Verification items for the finished model (mm, model axes). Face numbers are marked on the shaded views. A direction names the side the tool comes from. Round coordinates to 2 decimals unless told otherwise and drop trailing zeros. Write each loop counter-clockwise with the first axis right and the second up, starting at its lowest first coordinate (ties: lowest second). Pieces come first, ordered by that corner, then holes. Notation, with made-up numbers: (73, -29.75) - (129, -29.75) arc R16 ccw to (129, -18.75) - close; hole circle Ø8 at (-3, 11.25). An arc over 180 degrees is marked (long way). Answer as a JSON object with one key per item and string values. Group by question number.
1) Thickness scan on line 1 (X direction, y = 47, z = 80.5); line 2 (Y direction, x = 23, z = 63.5). Record the ranges inside material, lowest first.
2) Section check C-C (z = 52). Enter the section's corners in (x, y), then the cut area to 3 significant figures.
3) Section check B-B (y = 39.5). Enter the section's corners in (x, z), then the cut area to 3 significant figures.
4) Section check D-D (z = 25). Enter the section's corners in (x, y).
5) Section check A-A (x = 19.19). Enter the section's corners in (y, z).
6) Go/stop test with flat-tipped pins: pin 1 Ø4 at (x, z) = (2.5, 60.5) entering from -Y; pin 2 Ø6.5 at (x, z) = (47, 66.5) entering from -Y; pin 3 Ø3 at (x, y) = (46.5, -3.5) entering from -Z. Record where each tip stops, or that it passes through.
7) Set-up check for the marked faces 1 and 2: record each of +Z, -Z, +X, -X, +Y, -Y from which the full face is reachable in a straight line by a thin tool's end or side.
8) Mould release check, pull along X, two halves, no side actions. Record for the marked faces 3, 4 and 5: +X half, -X half, draft (parallel to the pull), parting line (faces both ways), or undercut.
```python
from build123d import *

# Parameters (mm, degrees)
BOSS_EXTRUDE1_DEPTH = 120
SKETCH2_W           = 20
SKETCH2_H           = 6
BOSS_EXTRUDE2_DEPTH = 6
SKETCH3_W           = 20
SKETCH3_H           = 6
BOSS_EXTRUDE3_DEPTH = 6
SKETCH4_R           = 1.6
CUT_EXTRUDE1_DEPTH  = 10


with BuildPart() as part:
    # Sketch1 → Boss-Extrude1 (new body)
    with BuildSketch(Plane.XY):
        Polygon((42.5, 0), (42.5, 50), (-42.5, 50), (-42.5, 0), (-48.5, 0), (-48.5, 56), (48.5, 56), (48.5, 0), align=None)
    extrude(amount=BOSS_EXTRUDE1_DEPTH)

    # Sketch2 → Boss-Extrude2 (add)
    with BuildSketch(Plane(origin=(48.5, 0, 0), x_dir=(0, 0, -1), z_dir=(1, 0, 0))):
        with Locations((-90, -3)):
            Rectangle(SKETCH2_W, SKETCH2_H)
        with Locations((-30, -3)):
            Rectangle(SKETCH2_W, SKETCH2_H)
    extrude(amount=-BOSS_EXTRUDE2_DEPTH)

    # Sketch3 → Boss-Extrude3 (add)
    with BuildSketch(Plane.ZY.offset(48.5)):
        with Locations((30, -3)):
            Rectangle(SKETCH3_W, SKETCH3_H)
        with Locations((90, -3)):
            Rectangle(SKETCH3_W, SKETCH3_H)
    extrude(amount=-BOSS_EXTRUDE3_DEPTH)

    # Sketch4 → Cut-Extrude1 (cut)
    with BuildSketch(Plane(origin=(0, 56, 0), x_dir=(1, 0, 0), z_dir=(0, 1, 0))):
        with Locations(Location((-23.905, -86.79842215, 0), (0, 0, 270))):
            Circle(SKETCH4_R)
        with Locations(Location((23.905, -86.79842215, 0), (0, 0, 270))):
            Circle(SKETCH4_R)
        with Locations(Location((-8.71, -35.65842215, 0), (0, 0, 270))):
            Circle(SKETCH4_R)
        with Locations(Location((19.19, -35.65842215, 0), (0, 0, 270))):
            Circle(SKETCH4_R)
    extrude(amount=-CUT_EXTRUDE1_DEPTH, mode=Mode.SUBTRACT)


solid = part.part
```
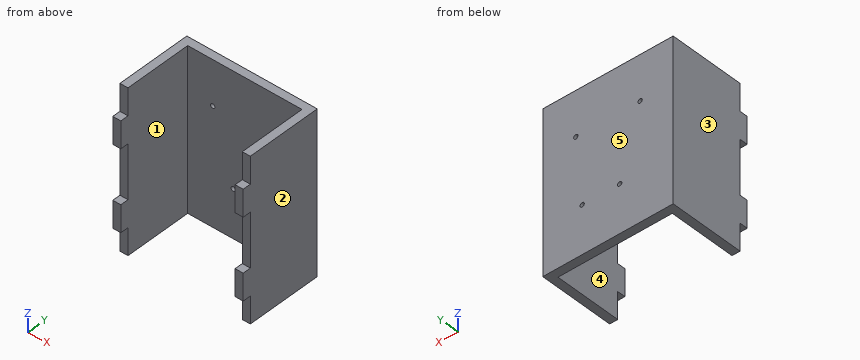
Returned:
{
 "1": {"line 1": "-48.5 to -42.5, 42.5 to 48.5", "line 2": "50 to 56"},
 "2": {"outline": "(-48.5, 0) - (-42.5, 0) - (-42.5, 50) - (42.5, 50) - (42.5, 0) - (48.5, 0) - (48.5, 56) - (-48.5, 56) - close", "area": "1,180 mm2"},
 "3": {"outline": "(-48.5, 0) - (-42.5, 0) - (-42.5, 120) - (-48.5, 120) - close; (42.5, 0) - (48.5, 0) - (48.5, 120) - (42.5, 120) - close", "area": "1,440 mm2"},
 "4": {"outline": "(-48.5, -6) - (-42.5, -6) - (-42.5, 50) - (42.5, 50) - (42.5, -6) - (48.5, -6) - (48.5, 56) - (-48.5, 56) - close"},
 "5": {"outline": "(50, 0) - (56, 0) - (56, 34.06) - (50, 34.06) - close; (50, 37.26) - (56, 37.26) - (56, 120) - (50, 120) - close"},
 "6": {"pin 1": "y = 50", "pin 2": "y = 0", "pin 3": "z = 20"},
 "7": {"face 1": "+Z, -Z, -Y", "face 2": "+Z, -Z, +X, +Y, -Y"},
 "8": {"face 3": "-X half", "face 4": "undercut", "face 5": "draft"}
}
